```python
from build123d import *

# Parameters (mm, degrees)
BOX019_W          = 8
BOX019_H          = 9
BOX019_DEPTH      = 8
FILLET027_R       = 7
FILLET028_R       = 4
CYLINDER_R        = 0.8
CYLINDER_DEPTH    = 10
CYLINDER029_R     = 8
CYLINDER029_DEPTH = 10
BOX018_W          = 22
BOX018_H          = 50
BOX018_DEPTH      = 8
FILLET025_R       = 2
BOX016_W          = 22
BOX016_H          = 50
BOX016_DEPTH      = 8
FILLET026_R       = 2
FILLET029_R       = 2


with BuildPart() as fillet028:
    # Box019 → Box019 (new body)
    with BuildSketch(Plane(origin=(-10, -30, 0), x_dir=(1, 0, 0), z_dir=(0, 0, 1))):
        with Locations((4, 4.5)):
            Rectangle(BOX019_W, BOX019_H)
    extrude(amount=BOX019_DEPTH)

    # Fillet027
    fillet027_edges = [fillet028.edges().sort_by_distance(p)[0] for p in [
        (-10, -25.5, 8),
    ]]
    fillet(fillet027_edges, radius=FILLET027_R)

    # Fillet028
    fillet028_edges = [fillet028.edges().sort_by_distance(p)[0] for p in [
        (-7.949747, -30, 5.949747),
        (-7.949747, -21, 5.949747),
    ]]
    fillet(fillet028_edges, radius=FILLET028_R)


with BuildPart() as obj1:
    # Cylinder → Cylinder (new body)
    with BuildSketch(Plane.XY):
        Circle(CYLINDER_R)
    extrude(amount=CYLINDER_DEPTH)


with BuildPart() as obj2:
    # Cylinder029 → Cylinder029 (new body)
    with BuildSketch(Plane.XY):
        Circle(CYLINDER029_R)
    extrude(amount=CYLINDER029_DEPTH)


with BuildPart() as fusion014:
    # Box018 → Box018 (new body)
    with BuildSketch(Plane(origin=(-11, -39, 1.5), x_dir=(1, 0, 0), z_dir=(0, 0, 1))):
        with Locations((11, 25)):
            Rectangle(BOX018_W, BOX018_H)
    extrude(amount=BOX018_DEPTH)

    # Cut008: cut obj2
    add(obj2.part, mode=Mode.SUBTRACT)

    # Fillet025
    fillet025_edges = [fusion014.edges().sort_by_distance(p)[0] for p in [
        (-8, 0, 1.5),
    ]]
    fillet(fillet025_edges, radius=FILLET025_R)

    # Fusion014: union obj1
    add(obj1.part)


with BuildPart() as obj3:
    # Box016 → Box016 (new body)
    with BuildSketch(Plane(origin=(-11, -39, 0), x_dir=(1, 0, 0), z_dir=(0, 0, 1))):
        with Locations((11, 25)):
            Rectangle(BOX016_W, BOX016_H)
    extrude(amount=BOX016_DEPTH)

    # Fillet026
    fillet026_edges = [obj3.edges().sort_by_distance(p)[0] for p in [
        (-11, -39, 4),
        (-11, 11, 4),
        (11, -39, 4),
        (11, 11, 4),
    ]]
    fillet(fillet026_edges, radius=FILLET026_R)

    # Cut009: cut Fusion014
    add(fusion014.part, mode=Mode.SUBTRACT)

    # Fillet029
    fillet029_edges = [obj3.edges().sort_by_distance(p)[0] for p in [
        (-8, 0, 8),
    ]]
    fillet(fillet029_edges, radius=FILLET029_R)

    # Fusion015: union Fillet028
    add(fillet028.part)


with BuildPart() as obj3_1:
    # Fusion015 placement: moved
    add(obj3.part.moved(Location((0, 84, 0))))


solid = obj3_1.part
```
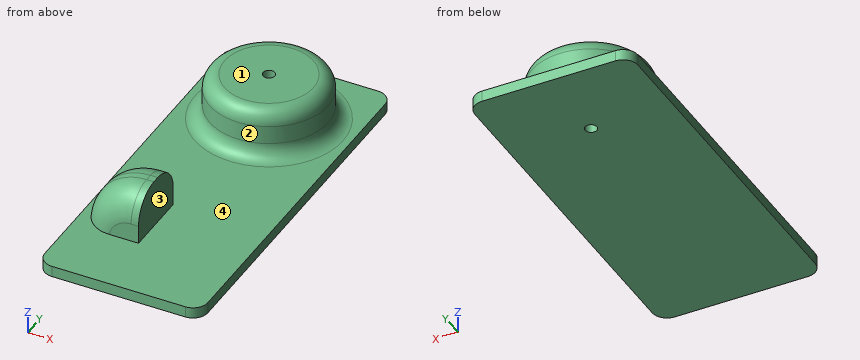
Work out the finished part from the listing and answer in its coordinate system (mm). Face numbers are marked on the shaded views. A direction names the side the tool comes from. Give positions to 0.01 mm unless a question says otherwise; leave off trailing zeros. Write each loop counter-clockwise with the first axis right and the second up, starting at its lowest first coordinate (ties: lowest second). Pieces come first, ordered by that corner, then holes. Notation, with made-up numbers: (-6, 20) - (49, 20) arc R28 cw to (49, 57) - close; hole circle Ø9 at (-31.5, 55). An arc over 180 degrees is marked (long way). Use one line per item in the form item = value.
1. A cutting plane is placed at A-A (y = 84). Write down the section's boundary in (x, z), and give its area (3 significant figures).
Filled in:
outline = (-11, 0) - (-0.8, 0) - (-0.8, 8) - (-6, 8) arc R2 ccw to (-8, 6) - (-8, 3.5) arc R2 cw to (-10, 1.5) - (-11, 1.5) - close; (0.8, 0) - (11, 0) - (11, 1.5) - (10, 1.5) arc R2 cw to (8, 3.5) - (8, 6) arc R2 ccw to (6, 8) - (0.8, 8) - close
area = 124 mm^2
2. Determine the mould class of the marked faces 3 and 4 for opening direction Y: released by +Y, released by -Y, zero draft, split by the parting line, or undercut.
Filled in:
face_3 = zero draft
face_4 = undercut
3. A cutting plane is placed at B-B (x = 0). Write down the section's boundary in (y, z), and give its area (3 significant figures).
Filled in:
outline = (45, 0) - (83.2, 0) - (83.2, 8) - (78, 8) arc R2 ccw to (76, 6) - (76, 3.5) arc R2 cw to (74, 1.5) - (45, 1.5) - close; (84.8, 0) - (95, 0) - (95, 1.5) - (94, 1.5) arc R2 cw to (92, 3.5) - (92, 6) arc R2 ccw to (90, 8) - (84.8, 8) - close
area = 166 mm^2
4. A cutting plane is placed at C-C (z = 7). State how many separate pieces and enclosed holes the cut face has, and give its area (3 significant figures).
Filled in:
separate_pieces = 2
enclosed_holes = 1
area = 211 mm^2
5. Each of these flat-tipped pins is pushed along its axis until it touches: pin 1 Ø1.3 at (x, z) = (-4.5, 3) entering from -Y; pin 2 Ø6 at (x, y) = (-8, 63.5) entering from +Z; pin 3 Ø1.5 at (x, z) = (-4, 7) entering from -Y. Where does it stop, or does it pass through?
Filled in:
pin_1 = 54
pin_2 = 6.55
pin_3 = 54.75
6. A cutting plane is placed at D-D (y = 49.5). Write down the section's boundary in (x, z).
Filled in:
outline = (-11, 0) - (11, 0) - (11, 1.5) - (-11, 1.5) - close
7. Consider L1, parallel to Y at x = 0, z = 5.5; L2, parallel to X at y = 84, z = 5.5; L3, parallel to Y at x = -6.25, z = 2.5. Determine where each line is inside the solid, lowest interval first.
Filled in:
L1 = 76 to 83.2, 84.8 to 92
L2 = -8 to -0.8, 0.8 to 8
L3 = 54.04 to 62.96, 78.59 to 89.41
8. For the marked faces 1 and 2, determine the directions among +Z, -Z, +X, -X, +Y, -Y from which every point of the face is accessible in a straight line to the end or side of a thin tool.
Filled in:
face_1 = +Z, +X, -X, +Y, -Y
face_2 = +Z
